```python
from build123d import *

# Parameters (mm, degrees)
SKETCH1_R                = 12
BOSS_EXTRUDE1_DEPTH      = 45
SKETCH2_R                = 18.5
BOSS_EXTRUDE2_DEPTH      = 5.5
SKETCH3_R                = 12
BOSS_EXTRUDE3_DEPTH      = 105
CUT_EXTRUDE1_DEPTH       = 42
BOSS_EXTRUDE4_REACH      = 160.792
BOSS_EXTRUDE4_END_RADIUS = 12
CUT_EXTRUDE2_START       = -102
CUT_EXTRUDE2_DEPTH       = 102
BOSS_EXTRUDE5_REACH      = 160.792
BOSS_EXTRUDE5_END_RADIUS = 12
SKETCH9_R                = 3.25
CUT_EXTRUDE3_DEPTH       = 30
CUT_EXTRUDE4_START       = -30
SKETCH10_R               = 3.25
CUT_EXTRUDE4_DEPTH       = 30
CHAMFER1_SIZE            = 1


with BuildPart() as part:
    # Sketch1 → Boss-Extrude1 (new body)
    with BuildSketch(Plane(origin=(0, 0, 0), x_dir=(1, 0, 0), z_dir=(0, 1, 0))):
        with Locations(Location((0, 0, 0), (0, 0, 90))):
            Circle(SKETCH1_R)
    extrude(amount=BOSS_EXTRUDE1_DEPTH)

    # Sketch2 → Boss-Extrude2 (add)
    with BuildSketch(Plane(origin=(0, 45, 0), x_dir=(1, 0, 0), z_dir=(0, 1, 0))):
        with Locations(Location((0, 0, 0), (0, 0, 270))):
            Circle(SKETCH2_R)
    extrude(amount=BOSS_EXTRUDE2_DEPTH)

    # Sketch3 → Boss-Extrude3 (add)
    with BuildSketch(Plane(origin=(0, 50.5, 0), x_dir=(1, 0, 0), z_dir=(0, 1, 0))):
        with Locations(Location((0, 0, 0), (0, 0, 90))):
            Circle(SKETCH3_R)
    extrude(amount=BOSS_EXTRUDE3_DEPTH)

    # Sketch4 → Cut-Extrude1 (cut)
    with BuildSketch(Plane.XZ):
        Polygon((-4, -12), (-4, -11.313708499), (-4, -7.813708499), (4, -7.813708499), (4, -12), align=None)
    extrude(amount=-CUT_EXTRUDE1_DEPTH, mode=Mode.SUBTRACT)

    # Boss-Extrude4: up to this cylinder (the profile starts inside it)
    boss_extrude4_end = Plane(origin=(0, 41.106528, 0), z_dir=(0, -1, 0)) * Cylinder(BOSS_EXTRUDE4_END_RADIUS, 346.584, mode=Mode.PRIVATE)
    # Sketch6 → Boss-Extrude4 (add, up to the surface)
    with BuildSketch(Plane(origin=(0, 0, -7.813708499), x_dir=(-1, 0, 0), z_dir=(0, 0, -1)), mode=Mode.PRIVATE) as boss_extrude4_sk1:
        with BuildLine():
            Line((-4, 42), (-4, 38))
            ThreePointArc((-4, 38), (-2.828427125, 40.828427125), (0, 42))
            Line((0, 42), (-4, 42))
        make_face()
    boss_extrude4_tool1 = extrude(boss_extrude4_sk1.sketch, amount=BOSS_EXTRUDE4_REACH, mode=Mode.PRIVATE) & boss_extrude4_end
    add(boss_extrude4_tool1.solids().sort_by_distance((3.106528, 41.106528, -7.813708))[0])
    # Sketch6 → Boss-Extrude4 (add, up to the surface)
    with BuildSketch(Plane(origin=(0, 0, -7.813708499), x_dir=(-1, 0, 0), z_dir=(0, 0, -1)), mode=Mode.PRIVATE) as boss_extrude4_sk2:
        with BuildLine():
            Line((4, 42), (0, 42))
            ThreePointArc((0, 42), (2.828427125, 40.828427125), (4, 38))
            Line((4, 38), (4, 42))
        make_face()
    boss_extrude4_tool2 = extrude(boss_extrude4_sk2.sketch, amount=BOSS_EXTRUDE4_REACH, mode=Mode.PRIVATE) & boss_extrude4_end
    add(boss_extrude4_tool2.solids().sort_by_distance((-3.106528, 41.106528, -7.813708))[0])

    # Sketch7 → Cut-Extrude2 (cut)
    with BuildSketch(Plane(origin=(0, 155.5, 0), x_dir=(1, 0, 0), z_dir=(0, 1, 0)).offset(CUT_EXTRUDE2_START)):
        with BuildLine():
            Line((4, 7.813708499), (4, 11.313708499))
            ThreePointArc((4, 11.313708499), (2.029223745, 11.827182716), (0, 12))
            ThreePointArc((0, 12), (-2.029223745, 11.827182716), (-4, 11.313708499))
            Line((-4, 11.313708499), (-4, 7.813708499))
            Line((-4, 7.813708499), (4, 7.813708499))
        make_face()
    extrude(amount=CUT_EXTRUDE2_DEPTH, mode=Mode.SUBTRACT)

    # Boss-Extrude5: up to this cylinder (the profile starts inside it)
    boss_extrude5_end = Plane(origin=(0, 54.393472, 0), z_dir=(0, -1, 0)) * Cylinder(BOSS_EXTRUDE5_END_RADIUS, 346.584, mode=Mode.PRIVATE)
    # Sketch8 → Boss-Extrude5 (add, up to the surface)
    with BuildSketch(Plane(origin=(0, 0, -7.813708499), x_dir=(-1, 0, 0), z_dir=(0, 0, -1)), mode=Mode.PRIVATE) as boss_extrude5_sk1:
        with BuildLine():
            Line((4, 53.5), (4, 57.5))
            ThreePointArc((4, 57.5), (2.828427125, 54.671572875), (0, 53.5))
            Line((0, 53.5), (4, 53.5))
        make_face()
    boss_extrude5_tool1 = extrude(boss_extrude5_sk1.sketch, amount=BOSS_EXTRUDE5_REACH, mode=Mode.PRIVATE) & boss_extrude5_end
    add(boss_extrude5_tool1.solids().sort_by_distance((-3.106528, 54.393472, -7.813708))[0])
    # Sketch8 → Boss-Extrude5 (add, up to the surface)
    with BuildSketch(Plane(origin=(0, 0, -7.813708499), x_dir=(-1, 0, 0), z_dir=(0, 0, -1)), mode=Mode.PRIVATE) as boss_extrude5_sk2:
        with BuildLine():
            Line((-4, 53.5), (0, 53.5))
            ThreePointArc((0, 53.5), (-2.828427125, 54.671572875), (-4, 57.5))
            Line((-4, 57.5), (-4, 53.5))
        make_face()
    boss_extrude5_tool2 = extrude(boss_extrude5_sk2.sketch, amount=BOSS_EXTRUDE5_REACH, mode=Mode.PRIVATE) & boss_extrude5_end
    add(boss_extrude5_tool2.solids().sort_by_distance((3.106528, 54.393472, -7.813708))[0])

    # Sketch9 → Cut-Extrude3 (cut)
    with BuildSketch(Plane.XZ):
        with Locations(Location((0, 0, 0), (0, 0, 270))):
            Circle(SKETCH9_R)
    extrude(amount=-CUT_EXTRUDE3_DEPTH, mode=Mode.SUBTRACT)

    # Sketch10 → Cut-Extrude4 (cut)
    with BuildSketch(Plane(origin=(0, 155.5, 0), x_dir=(1, 0, 0), z_dir=(0, 1, 0)).offset(CUT_EXTRUDE4_START)):
        with Locations(Location((0, 0, 0), (0, 0, 90))):
            Circle(SKETCH10_R)
    extrude(amount=CUT_EXTRUDE4_DEPTH, mode=Mode.SUBTRACT)

    # Chamfer1
    chamfer1_edges = [part.edges().sort_by_distance(p)[0] for p in [
        (0, 0, 12),
        (0, 155.5, 12),
    ]]
    chamfer(chamfer1_edges, length=CHAMFER1_SIZE)


solid = part.part
```
Geometry: final body of the model. Coordinates: model frame, mm. A direction names the side the tool comes from. Give positions to 0.01 mm unless a question says otherwise; leave off trailing zeros. Loops run counter-clockwise (first coordinate to the right, second up) from the corner with the lowest first, then second, coordinate; pieces in that order, holes last. Notation, with made-up numbers: (33.25, 75.25) - (87.25, 75.25) arc R35 cw to (87.25, 107.25) - close; hole circle Ø8 at (84.5, 40). An arc over 180 degrees is marked (long way). Answer as CSV lines item,"result". Start each with the question number.
(1) Section query B-B (y = 118). Output: boundary loops of the cut face in (x, z).
(2) Ray query, line 1 along X through (y, z) = (139.75, 0); line 2 along Y through (x, z) = (9, -12); line 3 along X through (y, z) = (59.5, -8). Return the intervals inside material, ascending. Write a range as [from, to].
(3) Pin query (flat end, axial travel): P1, Ø4, axis at x = 0, y = 126.5, coming from the -Z side; P2, Ø1, axis at y = 21.5, z = -9.5, coming from the +X side; P3, Ø12, axis at x = -11, y = 136.5, coming from the -Z side. Return the tip coordinate at first contact, or that it passes through.
(4) Mould query, pull axis Z, two halves, no side actions, for faces 4 (the face through (-0.44, 155.34, 11.15)), 5 (the face through (-1.978, 14.79, 2.579)), 6 (the face through (0, 21, -7.814)), 7 (the face through (0, 125.5, 0)). Classes: +Z half, -Z half, draft (parallel to the pull), parting line (faces both ways), or undercut.
(5) Section query A-A (z = 0). Output: boundary loops of the cut face in (x, y), and give its area (3 significant figures).
(6) Reachability of faces 1 (the face through (-12, 50.5, 4)), 2 (the face through (-4, 106, -10)), 3 (the face through (-12, 45, 4)) from +Z, -Z, +X, -X, +Y, -Y: full face, straight path, thin tool, end or side. Return the list, or none.
(7) Section query C-C (x = -13.5). Output: boundary loops of the cut face in (y, z), and give its area (3 significant figures).
Worked answers:
1,outline,"(-4, -11.31) - (-4, -7.81) - (4, -7.81) - (4, -11.31) arc R12 ccw (long way) to start"
2,line 1,"x = [-12, -3.25], [3.25, 12]"
2,line 2,"y = [45, 50.5]"
2,line 3,"x = [-8.94, -4], [4, 8.94]"
3,P1,"stops at z = -7.81"
3,P2,"stops at x = 7.94"
3,P3,"stops at z = -10.91"
4,face 4,"parting line"
4,face 5,"undercut"
4,face 6,"-Z half"
4,face 7,"undercut"
5,outline,"(-18.5, 45) - (-12, 45) - (-12, 1) - (-11, 0) - (-3.25, 0) - (-3.25, 30) - (3.25, 30) - (3.25, 0) - (11, 0) - (12, 1) - (12, 45) - (18.5, 45) - (18.5, 50.5) - (12, 50.5) - (12, 154.5) - (11, 155.5) - (3.25, 155.5) - (3.25, 125.5) - (-3.25, 125.5) - (-3.25, 155.5) - (-11, 155.5) - (-12, 154.5) - (-12, 50.5) - (-18.5, 50.5) - close"
5,area,"3,410 mm^2"
6,face 1,"+Y"
6,face 2,"-Z, +Y"
6,face 3,"-Y"
7,outline,"(45, -12.65) - (50.5, -12.65) - (50.5, 12.65) - (45, 12.65) - close"
7,area,"139 mm^2"
